from build123d import *

# Parameters (mm, degrees)
F0_R     = 32.703889
F1_DEPTH = 25.4
F2_R     = 5.08
F3_W     = 15.693672
F3_H     = 28.699555
F4_DEPTH = 25.4


with BuildPart() as f1:
    # F0 (on Front) → F1 (new body)
    with BuildSketch(Plane.XZ):
        Circle(F0_R)
    extrude(amount=F1_DEPTH)

    # F2
    f2_edges = [f1.edges().sort_by_distance(p)[0] for p in [
        (-32.703889, -25.4, 0),
    ]]
    fillet(f2_edges, radius=F2_R)

    # F3 (on face) → F4 (join)
    with BuildSketch(Plane(origin=(0, 0, 0), x_dir=(-1, 0, 0), z_dir=(0, 1, 0))):
        with Locations((-7.846836, -3.763053)):
            Rectangle(F3_W, F3_H)
    extrude(amount=F4_DEPTH)


solid = f1.part
Geometry check sheet. Reference: the model listing, model coordinates, mm. A direction names the side the tool comes from. Round coordinates to 2 decimals unless told otherwise and drop trailing zeros. Loops run counter-clockwise (first coordinate to the right, second up) from the corner with the lowest first, then second, coordinate; pieces in that order, holes last. Notation, with made-up numbers: (26.25, 25) -> (63.25, 25) arc R36 ccw to (63.25, 64) -> close; hole circle Ø7 at (-34.5, -23.75). An arc over 180 degrees is marked (long way). Answer as a JSON object with one key per item and string values. Group by question number.
Item 1: Cross-section at B-B, the plane y = -11.5. Record the cut outline in (x, z), plus the area to 3 significant figures.
Item 2: Depth check by flat-ended pin: pin 1 Ø2 at (x, y) = (21.5, -14.5) entering from -Z; pin 2 Ø1 at (x, z) = (9.5, -25) entering from +Y; pin 3 Ø4.5 at (x, y) = (11, 9.5) entering from +Z. Enter the tip coordinate at first touch or a pass-through.
Item 3: Set-up check for faces 1 (the face through (15.694, 13, -4)), 2 (the face through (0, 13, -4)), 3 (the face through (8, 13, 10.587)), 4 (the face through (8, 13, -18.113)): record each of +Z, -Z, +X, -X, +Y, -Y from which the full face is reachable in a straight line by a thin tool's end or side.
Item 4: Thickness scan on line 1 along Y through (x, z) = (-13, 5); line 2 along Z through (x, y) = (1, 19); line 3 along X through (y, z) = (-16.5, 0.5). Record the ranges inside material, lowest first.
Item 5: Cross-section at A-A, the plane z = 0. Record the cut outline in (x, y).
Item 6: Cross-section at C-C, the plane y = 1.5. Record the cut outline in (x, z).
Determined:
{
 "1": {"outline": "circle Ø65.41 at (0, 0)", "area": "3,360 mm²"},
 "2": {"pin 1": "stops at z = -25.48", "pin 2": "stops at y = 0", "pin 3": "stops at z = 10.59"},
 "3": {"face 1": "+Z, -Z, +X, +Y", "face 2": "+Z, -Z, -X, +Y", "face 3": "+Z, +X, -X, +Y", "face 4": "-Z, +X, -X, +Y"},
 "4": {"line 1": "y = -25.4 to 0", "line 2": "z = -18.11 to 10.59", "line 3": "x = -32.7 to 32.7"},
 "5": {"outline": "(-32.7, -20.32) arc R5.08 ccw to (-27.62, -25.4) -> (27.62, -25.4) arc R5.08 ccw to (32.7, -20.32) -> (32.7, 0) -> (15.69, 0) -> (15.69, 25.4) -> (0, 25.4) -> (0, 0) -> (-32.7, 0) -> close"},
 "6": {"outline": "(0, -18.11) -> (15.69, -18.11) -> (15.69, 10.59) -> (0, 10.59) -> close"}
}
